Input: part model. Units: mm. Frame: model coordinates. A direction names the side the tool comes from. Round coordinates to 2 decimals unless told otherwise and drop trailing zeros. Order: outer loops, then holes, each group sorted by start corner. A loop starts at its lowest first (then second) coordinate and runs counter-clockwise, first axis right, second up. Notation, with made-up numbers: (83, 52) -> (124, 52) arc R33 cw to (124, 90) -> close; hole circle Ø1 at (-11.75, 8.5). An arc over 180 degrees is marked (long way). Use a Markdown table: item, result.
from build123d import *

# Parameters (mm, degrees)
F1_DEPTH = 40
F2_R     = 12.5
F3_DEPTH = 60.001


with BuildPart() as f1:
    # F0 (on Front) → F1 (new body)
    with BuildSketch(Plane.XZ):
        with BuildLine():
            Line((-30, 95), (-30, 0))
            Line((-30, 0), (30, 0))
            Line((30, 0), (30, 95))
            Line((30, 95), (0.5, 95))
            Line((0.5, 95), (0.5, 76.489996))
            ThreePointArc((0.5, 76.489996), (0, 51.5), (-0.5, 76.489996))
            Line((-0.5, 76.489996), (-0.5, 95))
            Line((-0.5, 95), (-30, 95))
        make_face()
    extrude(amount=F1_DEPTH)

    # F2 (on face) → F3 (cut, through all)
    with BuildSketch(Plane.YZ.offset(30)):
        with Locations((-20, 25)):
            Circle(F2_R)
    extrude(amount=-F3_DEPTH, mode=Mode.SUBTRACT)


solid = f1.part
1) Cut plane C-C on z = 73. Return loops of the section in (x, y).
Results found:
| item | result |
|---|---|
| outline | (-30, -40) -> (-8.67, -40) -> (-8.67, 0) -> (-30, 0) -> close; (8.67, -40) -> (30, -40) -> (30, 0) -> (8.67, 0) -> close |
2) Cut plane D-D on x = 23. Return loops of the section in (y, z), and give its area (3 significant figures).
Results found:
| item | result |
|---|---|
| outline | (-40, 0) -> (0, 0) -> (0, 95) -> (-40, 95) -> close; hole circle Ø25 at (-20, 25) |
| area | 3,310 mm² |
3) Set-up query: faces 5 (the flat face through (0.5, -20, 86)), 6 (the flat face through (-15, -20, 95)). Return all of +Z, -Z, +X, -X, +Y, -Y with unobstructed straight access to the full face (end or side cutting, diameter ignored); none if empty.
Results found:
| item | result |
|---|---|
| face 5 | +Z, +Y, -Y |
| face 6 | +Z, +X, -X, +Y, -Y |
4) Pin query (flat end, axial travel): pin 1 Ø15 at (x, z) = (0, 64) entering from -Y; pin 2 Ø4 at (x, y) = (-23, -7) entering from -Z. Return the tip coordinate at first contact, or that it passes through.
Results found:
| item | result |
|---|---|
| pin 1 | passes through |
| pin 2 | stops at z = 0 |
5) Line query: L1, parallel to X at y = -26, z = 85.5; L2, parallel to X at y = -11, z = 64; L3, parallel to Z at x = 0, y = -20.5. Output: solid intervals per line, ascending. Write a range as [from, to].
Results found:
| item | result |
|---|---|
| L1 | x = [-30, -0.5], [0.5, 30] |
| L2 | x = [-30, -12.5], [12.5, 30] |
| L3 | z = [0, 12.51], [37.49, 51.5] |
6) Cut plane B-B on y = -20. Return loops of the section in (x, z).
Results found:
| item | result |
|---|---|
| outline | (-30, 0) -> (30, 0) -> (30, 12.5) -> (-30, 12.5) -> close; (-30, 37.5) -> (30, 37.5) -> (30, 95) -> (0.5, 95) -> (0.5, 76.49) arc R12.5 cw (long way) to (-0.5, 76.49) -> (-0.5, 95) -> (-30, 95) -> close |
7) Pull-direction query (X, two-part tool) for faces 1 (the flat face through (-30, -20, 48)), 2 (the cylindrical face through (0.54, -19.72, 51.51)), 3 (the flat face through (30, -20, 47)), 4 (the flat face through (0, 0, 48)); classes: +X half, -X half, draft (parallel to the pull), parting line (faces both ways), or undercut.
Results found:
| item | result |
|---|---|
| face 1 | -X half |
| face 2 | undercut |
| face 3 | +X half |
| face 4 | draft |
8) Cut plane A-A on x = -10. Return loops of the section in (y, z).
Results found:
| item | result |
|---|---|
| outline | (-40, 0) -> (0, 0) -> (0, 56.5) -> (-40, 56.5) -> close; (-40, 71.5) -> (0, 71.5) -> (0, 95) -> (-40, 95) -> close; hole circle Ø25 at (-20, 25) |
